Check sheet for the modelled part. Datum: model origin and axes. Units: mm. A direction names the side the tool comes from. Round coordinates to 2 decimals unless told otherwise and drop trailing zeros. Order: outer loops, then holes, each group sorted by start corner. A loop starts at its lowest first (then second) coordinate and runs counter-clockwise, first axis right, second up. Notation, with made-up numbers: (78, 28) -> (117, 28) arc R29 ccw to (117, 57) -> close; hole circle Ø5 at (3.5, 18.25). An arc over 180 degrees is marked (long way). Answer in a Markdown table with one row per item.
from build123d import *

# Parameters (mm, degrees)
F2_W      = 45.4
F2_H      = 31.4
F2_W_2    = 5.75
F2_H_2    = 5.75
F2_R      = 1.75
F2_W_3    = 29.5
F2_H_3    = 0.2
F2_W_4    = 0.2
F2_H_4    = 15.5
F3_DEPTH  = 1.2
F4_DEPTH  = 2
F5_W      = 45.4
F5_H      = 31.4
F5_W_2    = 41.4
F5_H_2    = 27.4
F6_DEPTH  = 4.2
F5_R      = 1.5
F7_DEPTH  = 6.2
F8_W      = 3.5
F8_H      = 1.5
F9_DEPTH  = 2
F10_W     = 8.4
F10_H     = 4.2
F11_DEPTH = 2
F12_W     = 9.4
F12_H     = 1.2
F13_DEPTH = 2.2


with BuildPart() as f3:
    # F2 (on Top) → F3 (new body)
    with BuildSketch(Plane.XY):
        with Locations((4.5342570215, -2.7560327426)):
            Rectangle(F2_W, F2_H)
        Polygon((-16.1657429785, 10.9439672574), (-10.2157429785, 10.9439672574), (19.2842570215, 10.9439672574), (25.2342570215, 10.9439672574), (25.2342570215, 4.9939672574), (25.2342570215, -10.5060327426), (25.2342570215, -16.4560327426), (19.2842570215, -16.4560327426), (-10.2157429785, -16.4560327426), (-16.1657429785, -16.4560327426), (-16.1657429785, -10.5060327426), (-16.1657429785, 4.9939672574), align=None, mode=Mode.SUBTRACT)
        with Locations((22.1592570215, 7.8689672574)):
            Rectangle(F2_W_2, F2_H_2)
        with Locations((22.0342570215, 7.7439672574)):
            Circle(F2_R, mode=Mode.SUBTRACT)
        with Locations((-13.0907429785, 7.8689672574)):
            Rectangle(F2_W_2, F2_H_2)
        with Locations((-12.9657429785, 7.7439672574)):
            Circle(F2_R, mode=Mode.SUBTRACT)
        with Locations((22.1592570215, -13.3810327426)):
            Rectangle(F2_W_2, F2_H_2)
        with Locations((22.0342570215, -13.2560327426)):
            Circle(F2_R, mode=Mode.SUBTRACT)
        with Locations((-13.0907429785, -13.3810327426)):
            Rectangle(F2_W_2, F2_H_2)
        with Locations((-12.9657429785, -13.2560327426)):
            Circle(F2_R, mode=Mode.SUBTRACT)
        with Locations((-12.9657429785, 7.7439672574)):
            Circle(F2_R)
        with Locations((22.0342570215, 7.7439672574)):
            Circle(F2_R)
        with Locations((22.0342570215, -13.2560327426)):
            Circle(F2_R)
        with Locations((-12.9657429785, -13.2560327426)):
            Circle(F2_R)
        with Locations((4.5342570215, -16.3560327426)):
            Rectangle(F2_W_3, F2_H_3)
        with Locations((4.5342570215, 10.8439672574)):
            Rectangle(F2_W_3, F2_H_3)
        with Locations((-16.0657429785, -2.7560327426)):
            Rectangle(F2_W_4, F2_H_4)
        with Locations((25.1342570215, -2.7560327426)):
            Rectangle(F2_W_4, F2_H_4)
        Polygon((-15.9657429785, -16.2560327426), (-15.9657429785, -10.5060327426), (-16.1657429785, -10.5060327426), (-16.1657429785, -16.4560327426), (-10.2157429785, -16.4560327426), (-10.2157429785, -16.2560327426), align=None)
        Polygon((-15.9657429785, 4.9939672574), (-15.9657429785, 10.7439672574), (-10.2157429785, 10.7439672574), (-10.2157429785, 10.9439672574), (-16.1657429785, 10.9439672574), (-16.1657429785, 4.9939672574), align=None)
        Polygon((25.2342570215, -10.5060327426), (25.0342570215, -10.5060327426), (25.0342570215, -16.2560327426), (19.2842570215, -16.2560327426), (19.2842570215, -16.4560327426), (25.2342570215, -16.4560327426), align=None)
        Polygon((19.2842570215, 10.9439672574), (19.2842570215, 10.7439672574), (25.0342570215, 10.7439672574), (25.0342570215, 4.9939672574), (25.2342570215, 4.9939672574), (25.2342570215, 10.9439672574), align=None)
    extrude(amount=F3_DEPTH)

    # F2 (on Top) → F4 (join)
    with BuildSketch(Plane.XY):
        with Locations((4.5342570215, -2.7560327426)):
            Rectangle(F2_W, F2_H)
        Polygon((-16.1657429785, 10.9439672574), (-10.2157429785, 10.9439672574), (19.2842570215, 10.9439672574), (25.2342570215, 10.9439672574), (25.2342570215, 4.9939672574), (25.2342570215, -10.5060327426), (25.2342570215, -16.4560327426), (19.2842570215, -16.4560327426), (-10.2157429785, -16.4560327426), (-16.1657429785, -16.4560327426), (-16.1657429785, -10.5060327426), (-16.1657429785, 4.9939672574), align=None, mode=Mode.SUBTRACT)
        Polygon((19.2842570215, 10.7439672574), (-10.2157429785, 10.7439672574), (-10.2157429785, 4.9939672574), (-15.9657429785, 4.9939672574), (-15.9657429785, -10.5060327426), (-10.2157429785, -10.5060327426), (-10.2157429785, -16.2560327426), (19.2842570215, -16.2560327426), (19.2842570215, -10.5060327426), (25.0342570215, -10.5060327426), (25.0342570215, 4.9939672574), (19.2842570215, 4.9939672574), align=None)
        with Locations((-13.0907429785, 7.8689672574)):
            Rectangle(F2_W_2, F2_H_2)
        with Locations((-12.9657429785, 7.7439672574)):
            Circle(F2_R, mode=Mode.SUBTRACT)
        with Locations((-13.0907429785, -13.3810327426)):
            Rectangle(F2_W_2, F2_H_2)
        with Locations((-12.9657429785, -13.2560327426)):
            Circle(F2_R, mode=Mode.SUBTRACT)
        with Locations((22.1592570215, -13.3810327426)):
            Rectangle(F2_W_2, F2_H_2)
        with Locations((22.0342570215, -13.2560327426)):
            Circle(F2_R, mode=Mode.SUBTRACT)
        with Locations((22.1592570215, 7.8689672574)):
            Rectangle(F2_W_2, F2_H_2)
        with Locations((22.0342570215, 7.7439672574)):
            Circle(F2_R, mode=Mode.SUBTRACT)
        with Locations((-12.9657429785, 7.7439672574)):
            Circle(F2_R)
        with Locations((-12.9657429785, -13.2560327426)):
            Circle(F2_R)
        with Locations((22.0342570215, -13.2560327426)):
            Circle(F2_R)
        with Locations((22.0342570215, 7.7439672574)):
            Circle(F2_R)
        with Locations((4.5342570215, 10.8439672574)):
            Rectangle(F2_W_3, F2_H_3)
        with Locations((4.5342570215, -16.3560327426)):
            Rectangle(F2_W_3, F2_H_3)
        with Locations((-16.0657429785, -2.7560327426)):
            Rectangle(F2_W_4, F2_H_4)
        with Locations((25.1342570215, -2.7560327426)):
            Rectangle(F2_W_4, F2_H_4)
        Polygon((-15.9657429785, 4.9939672574), (-15.9657429785, 10.7439672574), (-10.2157429785, 10.7439672574), (-10.2157429785, 10.9439672574), (-16.1657429785, 10.9439672574), (-16.1657429785, 4.9939672574), align=None)
        Polygon((-15.9657429785, -16.2560327426), (-15.9657429785, -10.5060327426), (-16.1657429785, -10.5060327426), (-16.1657429785, -16.4560327426), (-10.2157429785, -16.4560327426), (-10.2157429785, -16.2560327426), align=None)
        Polygon((25.2342570215, -10.5060327426), (25.0342570215, -10.5060327426), (25.0342570215, -16.2560327426), (19.2842570215, -16.2560327426), (19.2842570215, -16.4560327426), (25.2342570215, -16.4560327426), align=None)
        Polygon((19.2842570215, 10.9439672574), (19.2842570215, 10.7439672574), (25.0342570215, 10.7439672574), (25.0342570215, 4.9939672574), (25.2342570215, 4.9939672574), (25.2342570215, 10.9439672574), align=None)
    extrude(amount=-F4_DEPTH)

    # F5 (on face) → F6 (join)
    with BuildSketch(Plane.XY.offset(1.2)):
        with Locations((4.5342570215, -2.7560327426)):
            Rectangle(F5_W, F5_H)
        with Locations((4.5342570215, -2.7560327426)):
            Rectangle(F5_W_2, F5_H_2, mode=Mode.SUBTRACT)
    extrude(amount=F6_DEPTH)

    # F5 (on face) → F7 (join)
    with BuildSketch(Plane.XY.offset(1.2)):
        with Locations((-12.9657429785, 7.7439672574)):
            Circle(F5_R)
        with Locations((22.0342570215, 7.7439672574)):
            Circle(F5_R)
        with Locations((22.0342570215, -13.2560327426)):
            Circle(F5_R)
        with Locations((-12.9657429785, -13.2560327426)):
            Circle(F5_R)
    extrude(amount=F7_DEPTH)

    # F8 (on face) → F9 (cut, through all)
    with BuildSketch(Plane(origin=(-18.1657429785, 0, 0), x_dir=(0, -1, 0), z_dir=(-1, 0, 0))):
        with Locations((1.7560327426, 3.9)):
            Rectangle(F8_W, F8_H)
    extrude(amount=-F9_DEPTH, mode=Mode.SUBTRACT)

    # F10 (on face) → F11 (cut, through all)
    with BuildSketch(Plane.XZ.offset(18.4560327426)):
        with Locations((-3.9657429785, 3.3)):
            Rectangle(F10_W, F10_H)
    extrude(amount=-F11_DEPTH, mode=Mode.SUBTRACT)

    # F12 (on face) → F13 (cut, through all)
    with BuildSketch(Plane(origin=(0, 12.9439672574, 0), x_dir=(-1, 0, 0), z_dir=(0, 1, 0))):
        with Locations((0.9657429785, 0.6)):
            Rectangle(F12_W, F12_H)
    extrude(amount=-F13_DEPTH, mode=Mode.SUBTRACT)


solid = f3.part
Item 1: Depth check by flat-ended pin: P1, Ø2, axis at x = -4, z = 3, coming from the -Y side; P2, Ø15.5, axis at x = -2, y = -9.5, coming from the +Z side; P3, Ø2, axis at x = 2.5, z = 6, coming from the -Y side; P4, Ø4, axis at x = -11, y = -3, coming from the +Z side. Enter the tip coordinate at first touch or a pass-through.
Result sheet:
| item | result |
|---|---|
| P1 | stops at y = 10.94 |
| P2 | stops at z = 5.4 |
| P3 | stops at y = -18.46 |
| P4 | stops at z = 0 |
Item 2: Cross-section at C-C (y = 1). Record the boundary of the cut face in (x, z).
Result sheet:
| item | result |
|---|---|
| outline | (-18.17, -2) -> (27.23, -2) -> (27.23, 5.4) -> (25.23, 5.4) -> (25.23, 1.2) -> (25.03, 1.2) -> (25.03, 0) -> (-15.97, 0) -> (-15.97, 1.2) -> (-16.17, 1.2) -> (-16.17, 5.4) -> (-18.17, 5.4) -> close |
Item 3: Cross-section at B-B (z = 4). Record the boundary of the cut face in (x, y).
Result sheet:
| item | result |
|---|---|
| outline | (-18.17, -18.46) -> (-8.17, -18.46) -> (-8.17, -16.46) -> (-16.17, -16.46) -> (-16.17, -3.51) -> (-18.17, -3.51) -> close; (-18.17, -0.01) -> (-16.17, -0.01) -> (-16.17, 10.94) -> (25.23, 10.94) -> (25.23, -16.46) -> (0.23, -16.46) -> (0.23, -18.46) -> (27.23, -18.46) -> (27.23, 12.94) -> (-18.17, 12.94) -> close; circle Ø3 at (-12.97, -13.26); circle Ø3 at (-12.97, 7.74); circle Ø3 at (22.03, -13.26); circle Ø3 at (22.03, 7.74) |
Item 4: Mould release check, pull along Z, two halves, no side actions. Record for faces 1 (the flat face through (-13, -13, 7.4)), 2 (the flat face through (-1, 12, 1.2)), 3 (the flat face through (-10.216, -13, 1)): pulls with the +Z half, pulls with the -Z half, needs draft (parallel to the pull), parting line crosses it, or undercut.
Result sheet:
| item | result |
|---|---|
| face 1 | pulls with the +Z half |
| face 2 | undercut |
| face 3 | needs draft |
Item 5: Scan lines: line 1 (X direction, y = 6, z = 3.75); line 2 (Y direction, x = -13.5, z = 1); line 3 (X direction, y = -16.5, z = 2.75). Record each from-to range of solid material in increasing order. Write a range as [from, to].
Result sheet:
| item | result |
|---|---|
| line 1 | x = [-18.17, -16.17], [25.23, 27.23] |
| line 2 | y = [-18.46, -10.51], [4.99, 12.94] |
| line 3 | x = [-18.17, -8.17], [0.23, 27.23] |
Item 6: Cross-section at A-A (x = -4). Record the boundary of the cut face in (y, z), and give its area (3 significant figures).
Result sheet:
| item | result |
|---|---|
| outline | (-18.46, -2) -> (12.94, -2) -> (12.94, 0) -> (-16.26, 0) -> (-16.26, 1.2) -> (-18.46, 1.2) -> close; (10.94, 1.2) -> (12.94, 1.2) -> (12.94, 5.4) -> (10.94, 5.4) -> close |
| area | 73.8 mm^2 |
Item 7: Set-up check for faces 4 (the flat face through (-5.666, 12, 1)), 5 (the flat face through (0.234, -17, 3)), 6 (the flat face through (-17, -2, 3.15)), 7 (the flat face through (19.284, -13, 1)): record each of +Z, -Z, +X, -X, +Y, -Y from which the full face is reachable in a straight line by a thin tool's end or side.
Result sheet:
| item | result |
|---|---|
| face 4 | +Y |
| face 5 | +Z, -Y |
| face 6 | -X |
| face 7 | +Z |
Item 8: Cross-section at D-D (z = 0.5). Record the boundary of the cut face in (x, y).
Result sheet:
| item | result |
|---|---|
| outline | (-18.17, -18.46) -> (27.23, -18.46) -> (27.23, 12.94) -> (3.73, 12.94) -> (3.73, 10.74) -> (19.28, 10.74) -> (19.28, 4.99) -> (25.03, 4.99) -> (25.03, -10.51) -> (19.28, -10.51) -> (19.28, -16.26) -> (-10.22, -16.26) -> (-10.22, -10.51) -> (-15.97, -10.51) -> (-15.97, 4.99) -> (-10.22, 4.99) -> (-10.22, 10.74) -> (-5.67, 10.74) -> (-5.67, 12.94) -> (-18.17, 12.94) -> close |
